```python
from build123d import *

# Parameters (mm, degrees)
SKETCH2_R                              = 3.3
SKETCH2_R_2                            = 3
CUT_8XTIE_D6_6_2XDOWEL_D6_PCD128_DEPTH = 150
SKETCH3_R                              = 2.5
CUT_4XM6_MOTOR_TAPS_PCD90_DEPTH        = 12
SKETCH4_R                              = 6
CUT_COUPLING_ACCESS_D12_DEPTH          = 150


with BuildPart() as part:
    # Sketch1 → REV_Input_Housing_Motor_Adapter (revolve)
    with BuildSketch(Plane(origin=(0, 0, 0), x_dir=(1, 0, 0), z_dir=(0, 1, 0))):
        Polygon((16, -13), (22, -13), (22, -19), (50, -19), (50, -7.5), (70, -7.5), (70, -25), (40, -25), (40, -113), (53, -113), (53, -125), (35, -125), (35, -25), (22, -25), (22, -54), (16, -54), (16, -35), (13.5, -35), (13.5, -25), (16, -25), align=None)
    revolve(axis=Axis((0, 0, 150), (0, 0, -1)))

    # Sketch2 → CUT_8xTie_D6.6_2xDowel_D6_PCD128 (cut, symmetric)
    with BuildSketch(Plane.XY):
        with Locations(Location((64, 0, 0), (0, 0, 180))):
            Circle(SKETCH2_R)
        with Locations(Location((45.2548, 45.2548, 0), (0, 0, 180))):
            Circle(SKETCH2_R)
        with Locations(Location((0, 64, 0), (0, 0, 180))):
            Circle(SKETCH2_R)
        with Locations(Location((-45.2548, 45.2548, 0), (0, 0, 180))):
            Circle(SKETCH2_R)
        with Locations(Location((-64, 0, 0), (0, 0, 180))):
            Circle(SKETCH2_R)
        with Locations(Location((-45.2548, -45.2548, 0), (0, 0, 180))):
            Circle(SKETCH2_R)
        with Locations(Location((0, -64, 0), (0, 0, 180))):
            Circle(SKETCH2_R)
        with Locations(Location((45.2548, -45.2548, 0), (0, 0, 180))):
            Circle(SKETCH2_R)
        with Locations(Location((24.4917, 59.1283, 0), (0, 0, 180))):
            Circle(SKETCH2_R_2)
        with Locations(Location((-24.4917, -59.1283, 0), (0, 0, 180))):
            Circle(SKETCH2_R_2)
    extrude(amount=CUT_8XTIE_D6_6_2XDOWEL_D6_PCD128_DEPTH, both=True, mode=Mode.SUBTRACT)

    # Sketch3 → CUT_4xM6_Motor_Taps_PCD90 (cut)
    with BuildSketch(Plane.XY.offset(125)):
        with Locations((31.8198, 31.8198)):
            Circle(SKETCH3_R)
        with Locations((-31.8198, 31.8198)):
            Circle(SKETCH3_R)
        with Locations((-31.8198, -31.8198)):
            Circle(SKETCH3_R)
        with Locations((31.8198, -31.8198)):
            Circle(SKETCH3_R)
    extrude(amount=-CUT_4XM6_MOTOR_TAPS_PCD90_DEPTH, mode=Mode.SUBTRACT)

    # Sketch4 → CUT_Coupling_Access_D12 (cut, symmetric)
    with BuildSketch(Plane(origin=(0, 0, 0), x_dir=(1, 0, 0), z_dir=(0, 1, 0))):
        with Locations(Location((0, -65, 0), (0, 0, 90))):
            Circle(SKETCH4_R)
        with Locations(Location((0, -103, 0), (0, 0, 90))):
            Circle(SKETCH4_R)
    extrude(amount=CUT_COUPLING_ACCESS_D12_DEPTH, both=True, mode=Mode.SUBTRACT)


solid = part.part
```
Part model, mm, in its own coordinate system. A direction names the side the tool comes from. Give positions to 0.01 mm unless a question says otherwise; leave off trailing zeros. Loops run counter-clockwise (first coordinate to the right, second up) from the corner with the lowest first, then second, coordinate; pieces in that order, holes last. Notation, with made-up numbers: M 2,22.5 L 56,22.5 A20 ccw 56,35.5 Z; hole C 54,22 d10. An arc over 180 degrees is marked long. Return JSON: item names as keys, results as strings.
1) Pull direction Z, two halves, no side cores. Call faces 1 (the face through (-8.67, 39.05, 69.62)), 2 (the face through (-2.93, 13.18, 29.93)), 3 (the face through (7, 12, 25)): released by +Z, released by -Z, zero draft, split by the parting line, or undercut.
Calculated:
{"face 1": "undercut", "face 2": "zero draft", "face 3": "released by -Z"}
2) Saw through at C-C, the plane z = 111. List the corners of the cut face in (x, y).
Calculated:
{"outline": "C 0,0 d80; hole C 0,0 d70"}
3) Drill centre lines: line 1 (Z direction, x = 14, y = 50.5); line 2 (Y direction, x = 0, z = 21); line 3 (Z direction, x = 12, y = 39). Where is each one in solid material? Low to high.
Calculated:
{"line 1": "z = 7.5 to 25, 113 to 125", "line 2": "y = -70 to -67.3, -60.7 to -16, 16 to 60.7, 67.3 to 70", "line 3": "z = 19 to 25, 113 to 125"}
4) Saw through at A-A, the plane x = 64. List the corners of the cut face in (y, z), then the cut area to 3 significant figures.
Calculated:
{"outline": "M -28.35,7.5 L -3.3,7.5 L -3.3,25 L -28.35,25 Z; M 3.3,7.5 L 28.35,7.5 L 28.35,25 L 3.3,25 Z", "area": "877 mm2"}
5) Flat gauge pins, fed straight in: pin 1 Ø4 at (x, y) = (-45.25, -45.25) entering from +Z; pin 2 Ø5 at (x, z) = (32, 28) entering from +Y; pin 3 Ø10.5 at (x, y) = (-64, 0) entering from +Z; pin 4 Ø8 at (y, z) = (-37, 102) entering from +X. Where does each tip first touch, or does it go through?
Calculated:
{"pin 1": "passes through", "pin 2": "stops at y = 27.01", "pin 3": "stops at z = 25", "pin 4": "stops at x = 22.61"}
6) Saw through at D-D, the plane y = 0. Count the separate pieces of the cut face and the enclosed holes in it, then the cut area to 3 significant figures.
Calculated:
{"separate pieces": "4", "enclosed holes": "0", "area": "2,660 mm2"}
7) 3-axis set-ups, long thin cutter, end or side, ignore diameter. For faces 4 (the face through (30, 30, 25)), 5 (the face through (28, -45, 119)), 6 (the face through (47.69, -15.02, 13.17)), 7 (the face through (-44.539, -42.033, 16.127)), 8 (the face through (35, 11, 125)): which of +Z, -Z, +X, -X, +Y, -Y reach the whole face in a straight line?
Calculated:
{"face 4": "none", "face 5": "+Z", "face 6": "-Z", "face 7": "+Z, -Z", "face 8": "+Z, +X, -X, +Y, -Y"}
